The listing builds one solid part. Answer for the finished solid, in the listing's coordinates (mm). A direction names the side the tool comes from. Give positions to 0.01 mm unless a question says otherwise; leave off trailing zeros. Write each loop counter-clockwise with the first axis right and the second up, starting at its lowest first coordinate (ties: lowest second). Pieces come first, ordered by that corner, then holes. Notation, with made-up numbers: (15.25, -18.5) - (54.25, -18.5) arc R21 cw to (54.25, -14.5) - close; hole circle Ø3 at (44, 0). An arc over 180 degrees is marked (long way). Return JSON: item names as keys, results as strings.
from build123d import *

# Parameters (mm, degrees)
F1_DEPTH  = 25.4
F2_R      = 3.9624
F3_DEPTH  = 58.55227
F4_R      = 6.35
F5_DEPTH  = 6.096
F7_DEPTH  = 25.4
F8_DEPTH  = 25.4
F10_DEPTH = 66.549


with BuildPart() as f1:
    # F0 (on Front) → F1 (new body, symmetric)
    with BuildSketch(Plane.XZ):
        Polygon((91.112512, 0), (0, 0), (0, -12.7), (85.852, -12.7), (131.70327, -58.55127), (149.663782, -40.590758), (109.073024, 0), (100.092768, -8.980256), align=None)
    extrude(amount=F1_DEPTH, both=True)

    # F2 (on face) → F3 (cut, through all)
    with BuildSketch(Plane.XY):
        with Locations((15.748, 12.7)):
            Circle(F2_R)
        with Locations((15.748, -12.7)):
            Circle(F2_R)
        with Locations((69.596, 12.7)):
            Circle(F2_R)
        with Locations((69.596, -12.7)):
            Circle(F2_R)
    extrude(amount=-F3_DEPTH, mode=Mode.SUBTRACT)

    # F4 (on face) → F5 (cut)
    with BuildSketch(Plane(origin=(0, 0, -12.7), x_dir=(1, 0, 0), z_dir=(0, 0, -1))):
        with Locations((15.748, 12.7)):
            Circle(F4_R)
        with Locations((15.748, -12.7)):
            Circle(F4_R)
        with Locations((69.596, -12.7)):
            Circle(F4_R)
        with Locations((69.596, 12.7)):
            Circle(F4_R)
    extrude(amount=-F5_DEPTH, mode=Mode.SUBTRACT)

    # F6 (on face) → F7 (join)
    with BuildSketch(Plane(origin=(54.536512, 0, 54.536512), x_dir=(0.707107, 0, -0.707107), z_dir=(0.707107, 0, 0.707107))):
        with BuildLine():
            ThreePointArc((124.727698, 25.4), (130.973663, -0.030356), (124.485501, -25.4))
            Line((124.485501, -25.4), (134.530275, -25.4))
            Line((134.530275, -25.4), (134.530275, 25.4))
            Line((134.530275, 25.4), (124.727698, 25.4))
        make_face()
    extrude(amount=-F7_DEPTH)

    # F6 (on face) → F8 (cut)
    with BuildSketch(Plane(origin=(54.536512, 0, 54.536512), x_dir=(0.707107, 0, -0.707107), z_dir=(0.707107, 0, 0.707107))):
        with BuildLine():
            ThreePointArc((124.727698, 25.4), (130.973663, -0.030356), (124.485501, -25.4))
            Line((124.485501, -25.4), (134.530275, -25.4))
            Line((134.530275, -25.4), (134.530275, 25.4))
            Line((134.530275, 25.4), (124.727698, 25.4))
        make_face()
    extrude(amount=-F8_DEPTH, mode=Mode.SUBTRACT)

    # F9 (on face) → F10 (cut, through all)
    with BuildSketch(Plane(origin=(54.536512, 0, -54.536512), x_dir=(0, -1, 0), z_dir=(-0.707107, 0, 0.707107))):
        Polygon((9.652, 71.030275), (9.652, 77.126275), (-9.646871, 77.126275), (-9.646871, 71.030275), (-15.48255, 71.030275), (-15.48255, 64.426275), (16.01345, 64.426275), (16.01345, 71.030275), align=None)
    extrude(amount=-F10_DEPTH, mode=Mode.SUBTRACT)


solid = f1.part
Item 1: A cutting plane is placed at C-C on z = -27. Determine the outline of the cut face in (x, y), then the cut area to 3 significant figures.
Answer below:
{"outline": "(100.15, -25.4) - (136.07, -25.4) - (136.07, -9.65) - (127.45, -9.65) - (127.45, -16.01) - (118.11, -16.01) - (118.11, 15.48) - (127.45, 15.48) - (127.45, 9.65) - (136.07, 9.65) - (136.07, 25.4) - (100.15, 25.4) - close", "area": "1,360 mm²"}
Item 2: A cutting plane is placed at D-D on y = 12.7. Determine the outline of the cut face in (x, z), then the cut area to 3 significant figures.
Answer below:
{"outline": "(0, -12.7) - (9.4, -12.7) - (9.4, -6.6) - (11.79, -6.6) - (11.79, 0) - (0, 0) - close; (19.71, -6.6) - (22.1, -6.6) - (22.1, -12.7) - (63.25, -12.7) - (63.25, -6.6) - (65.63, -6.6) - (65.63, 0) - (19.71, 0) - close; (73.56, -6.6) - (75.95, -6.6) - (75.95, -12.7) - (85.85, -12.7) - (128.15, -55) - (137.13, -46.02) - (91.11, 0) - (73.56, 0) - close; (104.76, -4.31) - (141.8, -41.35) - (146.11, -37.04) - (109.07, 0) - close", "area": "1,980 mm²"}
Item 3: For faces 4 (the face through (104.646, 19.164, -4.427)), 5 (the face through (20, -13, -6.604)), 6 (the face through (120, -16.013, -25)), determine the directions among +Z, -Z, +X, -X, +Y, -Y from which every point of the face is accessible in a straight line to the end or side of a thin tool.
Answer below:
{"face 4": "+Z, +Y, -Y", "face 5": "-Z", "face 6": "none"}
Item 4: The mould has two halves that part along X. Classify faces 1 (the face through (82, -25.4, -10)), 2 (the face through (18.678, 18.334, -9.695)), 3 (the face through (128.08, 17.413, -19.007)): +X half, -X half, draft (parallel to the pull), parting line (faces both ways), or undercut.
Answer below:
{"face 1": "draft", "face 2": "undercut", "face 3": "+X half"}
Item 5: A cutting plane is placed at B-B on x = 69. Determine the outline of the cut face in (y, z), then the cut area to 3 significant figures.
Answer below:
{"outline": "(-25.4, -12.7) - (-19.02, -12.7) - (-19.02, -6.6) - (-16.62, -6.6) - (-16.62, 0) - (-25.4, 0) - close; (-8.78, -6.6) - (-6.38, -6.6) - (-6.38, -12.7) - (6.38, -12.7) - (6.38, -6.6) - (8.78, -6.6) - (8.78, 0) - (-8.78, 0) - close; (16.62, -6.6) - (19.02, -6.6) - (19.02, -12.7) - (25.4, -12.7) - (25.4, 0) - (16.62, 0) - close", "area": "388 mm²"}
Item 6: A cutting plane is placed at A-A on y = -12.7. Determine the outline of the cut face in (x, z), then the cut area to 3 significant figures.
Answer below:
{"outline": "(0, -12.7) - (9.4, -12.7) - (9.4, -6.6) - (11.79, -6.6) - (11.79, 0) - (0, 0) - close; (19.71, -6.6) - (22.1, -6.6) - (22.1, -12.7) - (63.25, -12.7) - (63.25, -6.6) - (65.63, -6.6) - (65.63, 0) - (19.71, 0) - close; (73.56, -6.6) - (75.95, -6.6) - (75.95, -12.7) - (85.85, -12.7) - (128.08, -54.92) - (137.06, -45.94) - (91.11, 0) - (73.56, 0) - close; (104.76, -4.31) - (141.73, -41.27) - (146.04, -36.96) - (109.07, 0) - close", "area": "1,970 mm²"}
Item 7: Consider L1, parallel to X at y = 12, z = -2; L2, parallel to Y at x = 123, z = -23; L3, parallel to Y at x = 109, z = -8. Determine where each line is inside the solid, lowest interval first.
Answer below:
{"L1": "x = 0 to 11.85, 19.65 to 65.7, 73.5 to 93.11, 107.07 to 111.07", "L2": "y = -25.4 to -16.01, 15.48 to 25.4", "L3": "y = -25.4 to -9.65, 9.65 to 25.4"}
Item 8: Flat-ended cylindrical pins translate along their axes: P1, Ø5, axis at x = 69.596, y = -12.7, coming from the +Z side; P2, Ø12.5, axis at x = 69.596, y = 12.7, coming from the -Z side; P3, Ø20.5, axis at x = 69.596, y = 12.7, coming from the +Z side; P4, Ø16.5, axis at x = 69.596, y = -12.7, coming from the -Z side. Find the tip coordinate at first contact, or state that the pin passes through.
Answer below:
{"P1": "passes through", "P2": "stops at z = -6.6", "P3": "stops at z = 0", "P4": "stops at z = -12.7"}
